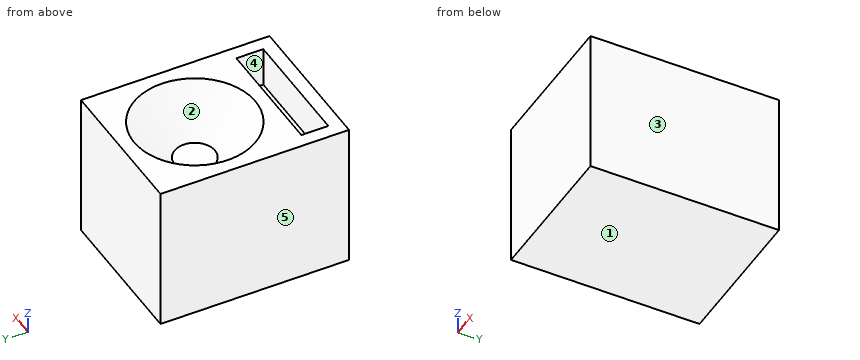
```python
from build123d import *

# Parameters (mm, degrees)
SKETCH1_W           = 558.8
SKETCH1_H           = 711.2
BOSS_EXTRUDE1_DEPTH = 558.8
SKETCH2_R           = 228.6
SKETCH2_W           = 457.2
SKETCH2_H           = 101.6
CUT_EXTRUDE1_DEPTH  = 152.4
CHAMFER1_SIZE       = 152.4


with BuildPart() as part:
    # Sketch1 → Boss-Extrude1 (new body)
    with BuildSketch(Plane.XY):
        with Locations((0, -76.2)):
            Rectangle(SKETCH1_W, SKETCH1_H)
    extrude(amount=BOSS_EXTRUDE1_DEPTH)

    # Sketch2 → Cut-Extrude1 (cut)
    with BuildSketch(Plane.XY.offset(558.8)):
        Circle(SKETCH2_R)
        with Locations((0, -330.2)):
            Rectangle(SKETCH2_W, SKETCH2_H)
    extrude(amount=-CUT_EXTRUDE1_DEPTH, mode=Mode.SUBTRACT)

    # Chamfer1
    chamfer1_edges = [part.edges().sort_by_distance(p)[0] for p in [
        (-228.6, 0, 406.4),
    ]]
    chamfer(chamfer1_edges, length=CHAMFER1_SIZE - 0.0001)  # a hair under: the kernel refuses the full size


solid = part.part
```
Input: part model. Units: mm. Frame: model coordinates. Face numbers are marked on the shaded views. A direction names the side the tool comes from. Give positions to 0.01 mm unless a question says otherwise; leave off trailing zeros. Order: outer loops, then holes, each group sorted by start corner. A loop starts at its lowest first (then second) coordinate and runs counter-clockwise, first axis right, second up. Notation, with made-up numbers: M 53.5,-6.75 L 68.5,-6.75 A6 cw 68.5,3.25 Z; hole C -13,3 d5. An arc over 180 degrees is marked long. One line per question, with ' | ' between items. Start each with the question number.
1. Access query for the marked faces 4 and 5. Directions: +Z, -Z, +X, -X, +Y, -Y. A direction counts if a zero-diameter tool reaches every point of the face in a straight line with its end or side. Return the directions, or none.
2. Section query B-B (z = 445.5). Return the cut outline in (x, y), and give its area (3 significant figures).
3. Pull-direction query (X, two-part tool) for the marked faces 1, 2 and 3; classes: released by +X, released by -X, zero draft, split by the parting line, or undercut.
4. Material intervals for probe 1 along Y at (x, z) = (-139, 490); probe 2 along Y at (x, z) = (0, 558); probe 3 along Z at (x, y) = (137, -356), sorted ascending. Write a range as [from, to].
Here are the results:
1) face 4: +Z | face 5: +Z, -Z, -X, +Y, -Y
2) outline: M -279.4,-431.8 L 279.4,-431.8 L 279.4,279.4 L -279.4,279.4 Z; hole M -228.6,-381 L 228.6,-381 L 228.6,-279.4 L -228.6,-279.4 Z; hole C 0,0 d230.6 | area: 309,000 mm²
3) face 1: zero draft | face 2: undercut | face 3: released by +X
4) probe 1: [-431.8, -381], [-279.4, -78.84], [78.84, 279.4] | probe 2: [-431.8, -381], [-279.4, -227.8], [227.8, 279.4] | probe 3: [0, 406.4]
